Answer from the drawing. Dimensions are ordinates in mm from the lowest x, y and z of the part. Coordinates: 2 decimals unless noted, no trailing zeros. Write each loop counter-clockwise with the first axis right and the second up, starting at its lowest first coordinate (ties: lowest second). Pieces come first, ordered by that corner, then holes. Notation, with made-up numbers: (34, 44.25) - (88, 44.25) arc R30 cw to (88, 71.25) - close; hole circle Ø10 at (49.5, 1.5). An arc over 180 degrees is marked (long way). Answer as a JSON object with one key per item and string values. Group by question number.
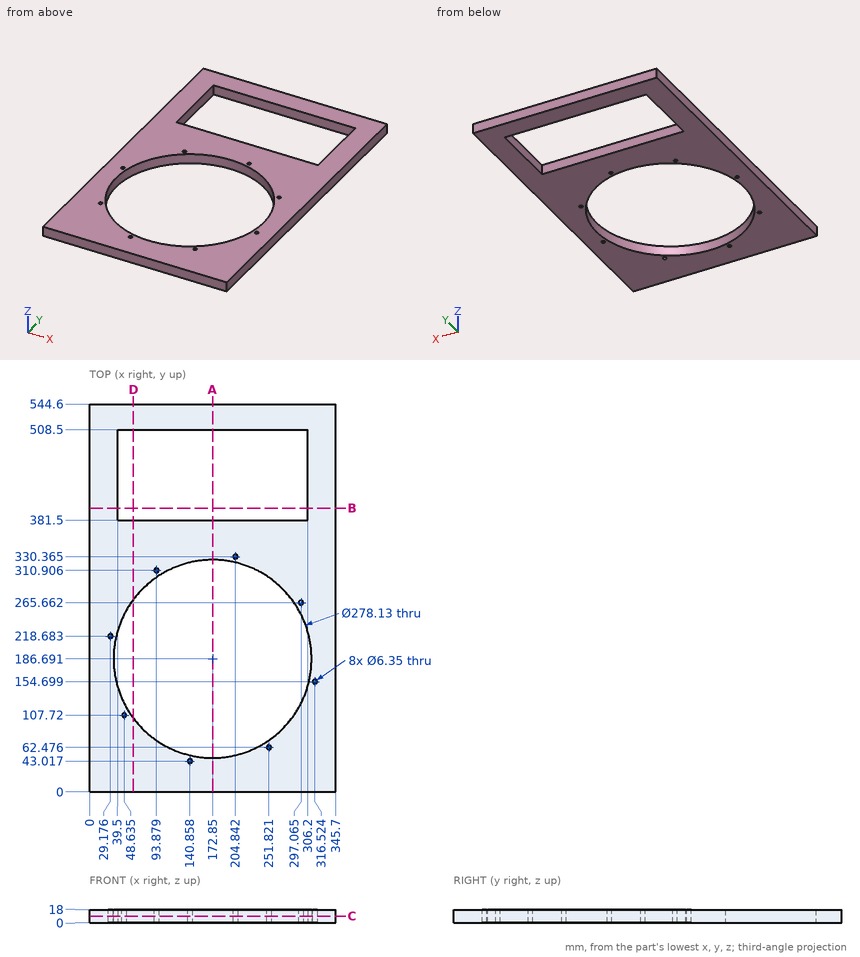
Q1. Section D-D on x = 61.5 is taken. Determine the outline of the cut face in (y, z), plus the area to 3 significant figures.
Q2. Section A-A on x = 172.85 is taken. Determine the outline of the cut face in (y, z).
Q3. Section C-C on z = 9.25 is taken. Count the separate pieces of the cut face and the enclosed holes in it, plus the area to 3 significant figures.
Q4. Section B-B on y = 398.5 is taken. Determine the outline of the cut face in (x, z), plus the area to 3 significant figures.
Q5. A flat-ended cylindrical pin translates along its axis: pin 1 Ø7.5 at (x, y) = (297.06, 265.66) entering from +Z. Find the tip coordinate at first contact, or state that the pin passes through.
Q6. Consider L1, parallel to Y at x = 223, z = 17.25; L2, parallel to Y at x = 132.5, z = 16; L3, parallel to X at y = 61.5, z = 4. Determine where each line is inside the solid, lowest interval first. Write a range as from..to.
Numbers:
{
 "1": {"outline": "(0, 0) - (103.38, 0) - (103.38, 18) - (0, 18) - close; (270, 0) - (381.5, 0) - (381.5, 18) - (270, 18) - close; (508.5, 0) - (544.6, 0) - (544.6, 18) - (508.5, 18) - close", "area": "4,520 mm²"},
 "2": {"outline": "(0, 0) - (47.63, 0) - (47.63, 18) - (0, 18) - close; (325.76, 0) - (381.5, 0) - (381.5, 18) - (325.76, 18) - close; (508.5, 0) - (544.6, 0) - (544.6, 18) - (508.5, 18) - close"},
 "3": {"separate pieces": "1", "enclosed holes": "10", "area": "93,400 mm²"},
 "4": {"outline": "(0, 0) - (39.5, 0) - (39.5, 18) - (0, 18) - close; (306.2, 0) - (345.7, 0) - (345.7, 18) - (306.2, 18) - close", "area": "1,420 mm²"},
 "5": {"pin 1": "stops at z = 18"},
 "6": {"L1": "y = 0..56.98, 316.4..381.5, 508.5..544.6", "L2": "y = 0..53.61, 319.77..381.5, 508.5..544.6", "L3": "x = 0..112.3, 233.4..248.8, 254.84..345.7"}
}
